Input: dimensioned drawing with shaded views. Units: mm. Origin: part minimum x, y, z. A direction names the side the tool comes from. Round coordinates to 2 decimals unless told otherwise and drop trailing zeros. Write each loop counter-clockwise with the first axis right and the second up, starting at its lowest first coordinate (ties: lowest second). Pieces come first, ordered by that corner, then holes. Notation, with made-up numbers: (-17.5, 6.5) -> (3.5, 6.5) arc R19 cw to (3.5, 19.5) -> close; hole circle Ø4 at (14.5, 76.5). An arc over 180 degrees is marked (long way). Use one line per item in the form item = value. Start each with the question number.
1. Reachability of the marked faces 5 and 6 from +Z, -Z, +X, -X, +Y, -Y: full face, straight path, thin tool, end or side. Return the list, or none.
2. Cut plane A-A, the plane x = 10. Return the cut outline in (y, z), plus the area to 3 significant figures.
3. Draft query along Z for the marked faces 1, 2, 3 and 4. Return one class per face: pulls with the +Z half, pulls with the -Z half, needs draft (parallel to the pull), parting line crosses it, or undercut.
4. Line query: L1, parallel to Y at x = 1, z = 10; L2, parallel to X at y = 2.25, z = 10; L3, parallel to X at y = 4.75, z = 14. Output: solid intervals per line, ascending.
5. Pin query (flat end, axial travel): pin 1 Ø5 at (y, z) = (10.5, 8) entering from +X; pin 2 Ø10 at (x, z) = (6, 14.5) entering from +Y; pin 3 Ø7 at (x, z) = (10, 10) entering from +Y. Return the tip coordinate at first contact, or that it passes through.
6. Cut plane D-D, the plane x = 14.75. Return the cut outline in (y, z).
7. Cut plane C-C, the plane z = 9.5. Return the cut outline in (x, y), plus the area to 3 significant figures.
8. Cut plane B-B, the plane y = 11.25. Return the cut outline in (x, z) (1 decimal), plus the area to 3 significant figures.
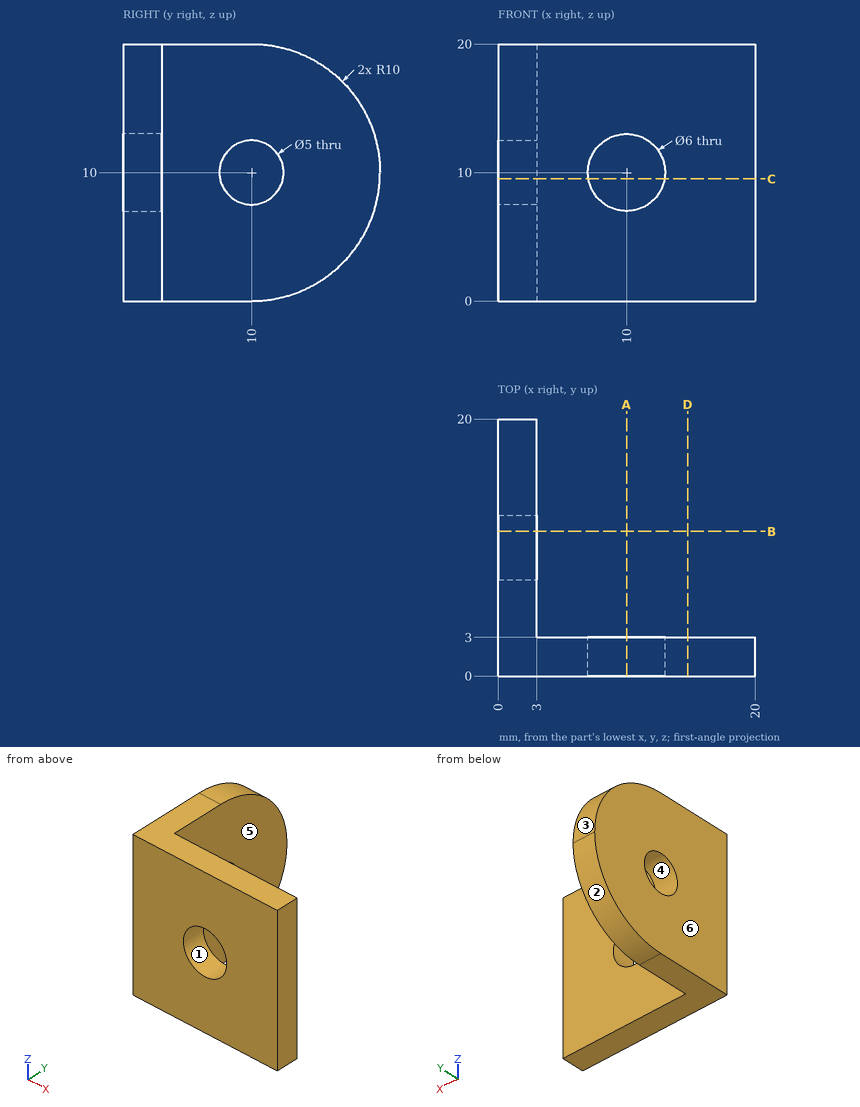
Outcome:
q1.face_5 = +Z, -Z, +X, +Y
q1.face_6 = +Z, -Z, -X, +Y, -Y
q2.outline = (0, 0) -> (3, 0) -> (3, 7) -> (0, 7) -> close; (0, 13) -> (3, 13) -> (3, 20) -> (0, 20) -> close
q2.area = 42.0 mm^2
q3.face_1 = undercut
q3.face_2 = pulls with the -Z half
q3.face_3 = pulls with the +Z half
q3.face_4 = undercut
q4.L1 = 0 to 7.5, 12.5 to 20
q4.L2 = 0 to 7, 13 to 20
q4.L3 = 0 to 3
q5.pin_1 = 3
q5.pin_2 = 19.99
q5.pin_3 = 3
q6.outline = (0, 0) -> (3, 0) -> (3, 20) -> (0, 20) -> close
q7.outline = (0, 0) -> (7.04, 0) -> (7.04, 3) -> (3, 3) -> (3, 7.55) -> (0, 7.55) -> close; (0, 12.45) -> (3, 12.45) -> (3, 19.99) -> (0, 19.99) -> close; (12.96, 0) -> (20, 0) -> (20, 3) -> (12.96, 3) -> close
q7.area = 78.5 mm^2
q8.outline = (0, 0.1) -> (3, 0.1) -> (3, 7.8) -> (0, 7.8) -> close; (0, 12.2) -> (3, 12.2) -> (3, 19.9) -> (0, 19.9) -> close
q8.area = 46.5 mm^2
